from build123d import *

# Parameters (mm, degrees)
F0_R     = 10
F1_DEPTH = 25


with BuildPart() as f1:
    # F0 (on Front) → F1 (new body)
    with BuildSketch(Plane.XZ):
        with BuildLine():
            ThreePointArc((107.5, 0), (102.879651, 11.847556), (91.458333, 17.43913))
            ThreePointArc((91.458333, 17.43913), (72.5, 0), (91.458333, -17.43913))
            ThreePointArc((91.458333, -17.43913), (102.879651, -11.847556), (107.5, 0))
        make_face()
        with Locations((90, 0)):
            Circle(F0_R, mode=Mode.SUBTRACT)
        with BuildLine():
            ThreePointArc((2.083333, 24.913043), (18.399502, 16.92508), (25, 0))
            ThreePointArc((25, 0), (18.399502, -16.92508), (2.083333, -24.913043))
            Line((2.083333, -24.913043), (91.458333, -17.43913))
            ThreePointArc((91.458333, -17.43913), (72.5, 0), (91.458333, 17.43913))
            Line((91.458333, 17.43913), (2.083333, 24.913043))
        make_face()
        with BuildLine():
            ThreePointArc((2.083333, -24.913043), (18.399502, -16.92508), (25, 0))
            ThreePointArc((25, 0), (18.399502, 16.92508), (2.083333, 24.913043))
            ThreePointArc((2.083333, 24.913043), (-25, 0), (2.083333, -24.913043))
        make_face()
        Circle(F0_R, mode=Mode.SUBTRACT)
    extrude(amount=F1_DEPTH)


solid = f1.part
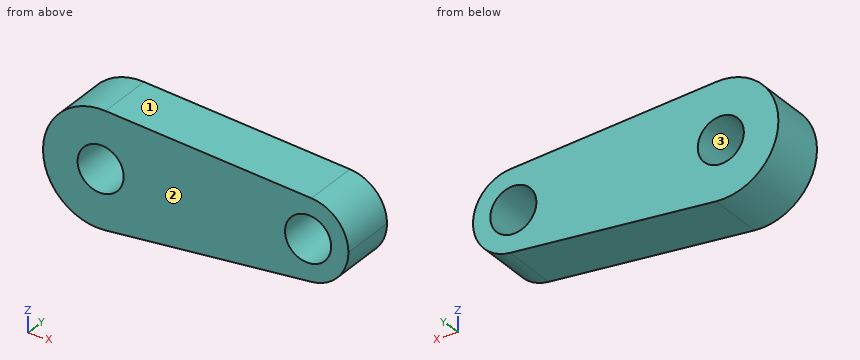
Input: part model. Units: mm. Frame: model coordinates. Face numbers are marked on the shaded views. Give positions to 0.01 mm unless a question says otherwise; leave off trailing zeros. Write each loop counter-clockwise with the first axis right and the second up, starting at its lowest first coordinate (ties: lowest second). Pieces come first, ordered by that corner, then holes. Notation, with made-up numbers: M -12,77 L 43,77 A17 cw 43,100 Z; hole C 26,29.5 d1. An arc over 180 degrees is marked long. Write item = value, one per line. Start each with the question number.
1) Material intervals for line 1 along X through (y, z) = (-5.5, 8); line 2 along X through (y, z) = (-2.75, -1); line 3 along Z through (x, y) = (90, -6.5), sorted ascending. Write a range as [from, to].
2) Cut plane C-C on z = -8. Return the cut outline in (x, y), then the cut area to 3 significant figures.
3) Cut plane A-A on x = 0. Return the cut outline in (y, z), then the cut area to 3 significant figures.
4) Cut plane D-D on x = 90. Return the cut outline in (y, z), then the cut area to 3 significant figures.
5) Draft query along X for the marked faces 1, 2 and 3. Return one class per face: +X half, -X half, draft (parallel to the pull), parting line (faces both ways), or undercut.
6) First-contact query: pin 1 Ø5 at (x, y) = (45, -18.5) entering from -Z; pin 2 Ø2 at (y, z) = (-16.5, 10) entering from +X; pin 3 Ø6 at (x, y) = (42, -7.5) entering from +Z; pin 4 Ø12 at (x, z) = (90, 0) entering from +Y. Flat tips, straight axial feed; report the tip coordinate or a pass-through.
7) Cut plane B-B on y = -15. Return the cut outline in (x, z), then the cut area to 3 significant figures.
Solved:
q1.line_1 = [-23.69, -6], [6, 84], [96, 105.56]
q1.line_2 = [-24.98, -9.95], [9.95, 80.05], [99.95, 107.47]
q1.line_3 = [-17.56, -10], [10, 17.56]
q2.outline = M -23.69,-25 L -6,-25 L -6,0 L -23.69,0 Z; M 6,-25 L 84,-25 L 84,0 L 6,0 Z; M 96,-25 L 105.56,-25 L 105.56,0 L 96,0 Z
q2.area = 2,630 mm2
q3.outline = M -25,-25 L 0,-25 L 0,-10 L -25,-10 Z; M -25,10 L 0,10 L 0,25 L -25,25 Z
q3.area = 750 mm2
q4.outline = M -25,-17.56 L 0,-17.56 L 0,-10 L -25,-10 Z; M -25,10 L 0,10 L 0,17.56 L -25,17.56 Z
q4.area = 378 mm2
q5.face_1 = +X half
q5.face_2 = draft
q5.face_3 = undercut
q6.pin_1 = -21.53
q6.pin_2 = 105.01
q6.pin_3 = 21.83
q6.pin_4 = through
q7.outline = M 2.08,-24.91 L 91.46,-17.44 A17.5 ccw 91.46,17.44 L 2.08,24.91 A25 ccw long Z; hole C 0,0 d20; hole C 90,0 d20
q7.area = 4,670 mm2
